```python
from build123d import *

# Parameters (mm, degrees)
SKETCH1_W               = 20
SKETCH1_H               = 20
BOSS_EXTRUDE2_DEPTH     = 12
BOSS_EXTRUDE3_DEPTH     = 4
SKETCH3_R               = 2.6
CUT_EXTRUDE1_DEPTH      = 7
BOSS_EXTRUDE4_DEPTH     = 40
BODY_MOVE_COPY1_ANGLE   = 45
CUT_EXTRUDE2_DEPTH      = 40
CUT_EXTRUDE2_DEPTH_BACK = 40
CUT_EXTRUDE3_DEPTH      = 40
CUT_EXTRUDE3_DEPTH_BACK = 40
CUT_EXTRUDE4_DEPTH      = 40
CUT_EXTRUDE4_DEPTH_BACK = 40
CUT_EXTRUDE7_DEPTH      = 40
CUT_EXTRUDE7_DEPTH_BACK = 40
BODY_MOVE_COPY2_ANGLE   = 45
SKETCH11_W              = 10
SKETCH11_H              = 10
CUT_EXTRUDE8_DEPTH      = 10
CUT_EXTRUDE9_DEPTH      = 17


with BuildPart() as part:
    # Sketch1 → Boss-Extrude2 (new body)
    with BuildSketch(Plane(origin=(0, 0, 0), x_dir=(1, 0, 0), z_dir=(0, 1, 0))):
        Rectangle(SKETCH1_W, SKETCH1_H)
    extrude(amount=-BOSS_EXTRUDE2_DEPTH)

    # Sketch2 → Boss-Extrude3 (add)
    with BuildSketch(Plane(origin=(0, 0, 0), x_dir=(1, 0, 0), z_dir=(0, 1, 0))):
        with BuildLine():
            Line((11.25, -5.593145751), (36.062445841, -30.405591591))
            ThreePointArc((36.062445841, -30.405591591), (38.890872965, -38.890872965), (30.405591591, -36.062445841))
            Line((30.405591591, -36.062445841), (5.593145751, -11.25))
            Line((5.593145751, -11.25), (-5.593145751, -11.25))
            Line((-5.593145751, -11.25), (-30.405591591, -36.062445841))
            ThreePointArc((-30.405591591, -36.062445841), (-38.890872965, -38.890872965), (-36.062445841, -30.405591591))
            Line((-36.062445841, -30.405591591), (-11.25, -5.593145751))
            Line((-11.25, -5.593145751), (-11.25, 5.593145751))
            Line((-11.25, 5.593145751), (-36.062445841, 30.405591591))
            ThreePointArc((-36.062445841, 30.405591591), (-38.890872965, 38.890872965), (-30.405591591, 36.062445841))
            Line((-30.405591591, 36.062445841), (-5.593145751, 11.25))
            Line((-5.593145751, 11.25), (5.593145751, 11.25))
            Line((5.593145751, 11.25), (30.405591591, 36.062445841))
            ThreePointArc((30.405591591, 36.062445841), (38.890872965, 38.890872965), (36.062445841, 30.405591591))
            Line((36.062445841, 30.405591591), (11.25, 5.593145751))
            Line((11.25, 5.593145751), (11.25, -5.593145751))
        make_face()
    extrude(amount=BOSS_EXTRUDE3_DEPTH)

    # Sketch3 → Cut-Extrude1 (cut)
    with BuildSketch(Plane(origin=(0, 0, 0), x_dir=(1, 0, 0), z_dir=(0, 1, 0))):
        with Locations(Location((-35.355339059, -35.355339059, 0), (0, 0, 270))):
            Circle(SKETCH3_R)
        with Locations(Location((-35.355339059, 35.355339059, 0), (0, 0, 270))):
            Circle(SKETCH3_R)
        with Locations(Location((35.355339059, 35.355339059, 0), (0, 0, 270))):
            Circle(SKETCH3_R)
        with Locations(Location((35.355339059, -35.355339059, 0), (0, 0, 270))):
            Circle(SKETCH3_R)
    extrude(amount=CUT_EXTRUDE1_DEPTH, mode=Mode.SUBTRACT)

    # Sketch4 → Boss-Extrude4 (add)
    with BuildSketch(Plane(origin=(0, 4, 0), x_dir=(1, 0, 0), z_dir=(0, 1, 0))):
        Polygon((-35.355339059, -31.112698372), (-31.112698372, -35.355339059), (-7.007359313, -11.25), (7.007359313, -11.25), (31.112698372, -35.355339059), (35.355339059, -31.112698372), (11.25, -7.007359313), (11.25, 7.007359313), (35.355339059, 31.112698372), (31.112698372, 35.355339059), (7.007359313, 11.25), (-7.007359313, 11.25), (-31.112698372, 35.355339059), (-35.355339059, 31.112698372), (-11.25, 7.007359313), (-11.25, -7.007359313), align=None)
    extrude(amount=BOSS_EXTRUDE4_DEPTH)


with BuildPart() as part_1:
    # Body-Move/Copy1: moved
    add(part.part.rotate(Axis((0, 0, 0), (0, 1, 0)), BODY_MOVE_COPY1_ANGLE))

    # Sketch6 → Cut-Extrude2 (cut, two sides: drawn at the far end of the back side and taken through both)
    with BuildSketch(Plane(origin=(0, 0, 0), x_dir=(0, 0, -1), z_dir=(1, 0, 0)).offset(-CUT_EXTRUDE2_DEPTH_BACK)):
        Polygon((-12.909902577, 44), (-47, 4), (-47, 44), align=None)
        Polygon((47, 44), (12.909902577, 44), (47, 4), align=None)
    extrude(amount=CUT_EXTRUDE2_DEPTH + CUT_EXTRUDE2_DEPTH_BACK, mode=Mode.SUBTRACT)

    # Sketch7 → Cut-Extrude3 (cut, two sides: drawn at the far end of the back side and taken through both)
    with BuildSketch(Plane.XY.offset(-CUT_EXTRUDE3_DEPTH_BACK)):
        Polygon((-47, 44), (-12.909902577, 44), (-47, 4), align=None)
        Polygon((47, 4), (47, 44), (12.909902577, 44), align=None)
    extrude(amount=CUT_EXTRUDE3_DEPTH + CUT_EXTRUDE3_DEPTH_BACK, mode=Mode.SUBTRACT)

    # Sketch8 → Cut-Extrude4 (cut, two sides: drawn at the far end of the back side and taken through both)
    with BuildSketch(Plane.XY.offset(-CUT_EXTRUDE4_DEPTH_BACK)):
        Polygon((-23.135931904, 6.857449794), (-29.954951288, 19), (-16.316912521, 35.002346486), (-16.316912521, 9), (-16.316912521, 6.857449794), align=None)
        Polygon((-29.954951288, 6.857449794), (-33.876748144, 13.840948819), (-34.065426963, 14.176927043), (-40.303469276, 6.857449794), align=None)
        Polygon((16.316912521, 9), (16.316912521, 35.002346486), (29.954951288, 19), (23.135931904, 6.857449794), (16.316912521, 6.857449794), align=None)
        Polygon((29.954951288, 6.857449794), (33.876748144, 13.840948819), (34.065426963, 14.176927043), (40.303469276, 6.857449794), align=None)
    extrude(amount=CUT_EXTRUDE4_DEPTH + CUT_EXTRUDE4_DEPTH_BACK, mode=Mode.SUBTRACT)

    # Sketch9 → Cut-Extrude7 (cut, two sides: drawn at the far end of the back side and taken through both)
    with BuildSketch(Plane(origin=(0, 0, 0), x_dir=(0, 0, -1), z_dir=(1, 0, 0)).offset(-CUT_EXTRUDE7_DEPTH_BACK)):
        Polygon((-23.135931904, 6.857449794), (-29.954951288, 19), (-16.316912521, 35.002346486), (-16.316912521, 9), (-16.316912521, 6.857449794), align=None)
        Polygon((-29.954951288, 6.857449794), (-33.876748144, 13.840948819), (-34.065426963, 14.176927043), (-40.303469276, 6.857449794), align=None)
        Polygon((16.316912521, 9), (16.316912521, 35.002346486), (29.954951288, 19), (23.135931904, 6.857449794), (16.316912521, 6.857449794), align=None)
        Polygon((29.954951288, 6.857449794), (33.876748144, 13.840948819), (34.065426963, 14.176927043), (40.303469276, 6.857449794), align=None)
    extrude(amount=CUT_EXTRUDE7_DEPTH + CUT_EXTRUDE7_DEPTH_BACK, mode=Mode.SUBTRACT)


with BuildPart() as part_2:
    # Body-Move/Copy2: moved
    add(part_1.part.rotate(Axis((0, 0, 0), (0, 1, 0)), BODY_MOVE_COPY2_ANGLE))

    # Sketch11 → Cut-Extrude8 (cut)
    with BuildSketch(Plane(origin=(0, 44, 0), x_dir=(1, 0, 0), z_dir=(0, 1, 0))):
        Rectangle(SKETCH11_W, SKETCH11_H)
    extrude(amount=-CUT_EXTRUDE8_DEPTH, mode=Mode.SUBTRACT)

    # Sketch12 → Cut-Extrude9 (cut)
    with BuildSketch(Plane(origin=(0, 4, 0), x_dir=(1, 0, 0), z_dir=(0, 1, 0))):
        Polygon((-35.355339059, -31.112698372), (-31.112698372, -35.355339059), (-30.264170235, -34.506810922), (-34.506810922, -30.264170235), align=None)
        Polygon((-30.264170235, 34.506810922), (-31.112698372, 35.355339059), (-35.355339059, 31.112698372), (-34.506810922, 30.264170235), align=None)
        Polygon((34.506810922, 30.264170235), (35.355339059, 31.112698372), (31.112698372, 35.355339059), (30.264170235, 34.506810922), align=None)
        Polygon((30.264170235, -34.506810922), (31.112698372, -35.355339059), (35.355339059, -31.112698372), (34.506810922, -30.264170235), align=None)
    extrude(amount=CUT_EXTRUDE9_DEPTH, mode=Mode.SUBTRACT)


solid = part_2.part
```
Input: part model. Units: mm. Frame: model coordinates. A direction names the side the tool comes from. Give positions to 0.01 mm unless a question says otherwise; leave off trailing zeros. Write each loop counter-clockwise with the first axis right and the second up, starting at its lowest first coordinate (ties: lowest second). Pieces come first, ordered by that corner, then holes. Notation, with made-up numbers: (18, -30) - (73, -30) arc R15 ccw to (73, -20) - close; hole circle Ø8 at (-8, -38.5). An arc over 180 degrees is marked (long way). Write item = value, one per line. Start each with the question number.
1. Section query A-A, the plane x = -1. Output: boundary loops of the cut face in (y, z).
2. Section query D-D, the plane z = -28.5. Output: boundary loops of the cut face in (x, y).
3. Ray query, L1, parallel to Z at x = 33.5, y = 2.5; L2, parallel to Z at x = -15.5, y = 31; L3, parallel to X at y = -6, z = 0. Return the intervals inside material, ascending.
4. Section query C-C, the plane y = 29. Count the separate pieces of the cut face and the enclosed holes in it, then the cut area to 3 significant figures.
5. First-contact query: pin 1 Ø6 at (x, y) = (26, 22.5) entering from -Z; pin 2 Ø4 at (y, z) = (11, -12) entering from -X; pin 3 Ø2.5 at (x, z) = (16, -14) entering from +Y. Flat tips, straight axial feed; report the tip coordinate or a pass-through.
6. Section query B-B, the plane z = 17. Output: boundary loops of the cut face in (x, y), then the cut area to 3 significant figures.
7. Access query for faces 4 (the flat face through (-16.3, 27.1, -16.3)), 5 (the flat face through (-18.8, 14.83, 23.04)), 6 (the flat face through (0, -6, -10)). Directions: +Z, -Z, +X, -X, +Y, -Y. A direction counts if a zero-diameter tool reaches every point of the face in a straight line with its end or side. Return the directions, or none.
8. Mould query, pull axis X, two halves, no side actions, for faces 1 (the flat face through (-14, 6.857, -14)), 2 (the flat face through (23.83, 1.972, -18.173)), 3 (the flat face through (-9, 0, 12)). Classes: released by +X, released by -X, zero draft, split by the parting line, or undercut.
Check sheet entries:
q1.outline = (-12, -10) - (0, -10) - (0, -11.25) - (44, -11.25) - (44, -5) - (34, -5) - (34, 5) - (44, 5) - (44, 11.25) - (0, 11.25) - (0, 10) - (-12, 10) - close
q2.outline = (-34.16, 0) - (-22.84, 0) - (-22.84, 4) - (-24.26, 4) - (-24.26, 6.86) - (-28.5, 6.86) - (-24.26, 10.38) - (-24.26, 15.38) - (-32.74, 8.34) - (-32.74, 4) - (-34.16, 4) - close; (22.84, 0) - (34.16, 0) - (34.16, 4) - (32.74, 4) - (32.74, 8.34) - (24.26, 15.38) - (24.26, 10.38) - (28.5, 6.86) - (24.26, 6.86) - (24.26, 4) - (22.84, 4) - close
q3.L1 = -40 to -37.18, -33.53 to -27.84, 27.84 to 33.53, 37.18 to 40
q3.L2 = -18.43 to -12.4, 12.4 to 18.43
q3.L3 = -10 to 10
q4.separate_pieces = 5
q4.enclosed_holes = 0
q4.area = 654 mm2
q5.pin_1 = -22.87
q5.pin_2 = -13.08
q5.pin_3 = 35.72
q6.outline = (-22.66, 0) - (-11.34, 0) - (-11.34, 4) - (-12.76, 4) - (-12.76, 6.86) - (-15.72, 6.86) - (-21.24, 13.81) - (-21.24, 4) - (-22.66, 4) - close; (-21.24, 22.42) - (-12.76, 29.46) - (-12.76, 34.46) - (-21.24, 27.42) - close; (11.34, 0) - (22.66, 0) - (22.66, 4) - (21.24, 4) - (21.24, 13.81) - (15.72, 6.86) - (12.76, 6.86) - (12.76, 4) - (11.34, 4) - close; (12.76, 29.46) - (21.24, 22.42) - (21.24, 27.42) - (12.76, 34.46) - close
q6.area = 262 mm2
q7.face_4 = none
q7.face_5 = +Z, +Y
q7.face_6 = -Z, +X, -X, -Y
q8.face_1 = undercut
q8.face_2 = released by +X
q8.face_3 = zero draft
